from build123d import *

# Parameters (mm, degrees)
F0_R     = 2.25
F1_DEPTH = 1.5


with BuildPart() as f1:
    # F0 (on Top) → F1 (new body)
    with BuildSketch(Plane.XY):
        with BuildLine():
            Line((52.9, 74.5), (-52.9, 74.5))
            ThreePointArc((-52.9, 74.5), (-53.465685, 74.265685), (-53.7, 73.7))
            Line((-53.7, 73.7), (-53.7, 68.7))
            ThreePointArc((-53.7, 68.7), (-56.248171, 62.548171), (-62.4, 60))
            Line((-62.4, 60), (-73.7, 60))
            ThreePointArc((-73.7, 60), (-74.265685, 59.765685), (-74.5, 59.2))
            Line((-74.5, 59.2), (-74.5, -59.2))
            ThreePointArc((-74.5, -59.2), (-74.265685, -59.765685), (-73.7, -60))
            Line((-73.7, -60), (-62.4, -60))
            ThreePointArc((-62.4, -60), (-56.248171, -62.548171), (-53.7, -68.7))
            Line((-53.7, -68.7), (-53.7, -73.7))
            ThreePointArc((-53.7, -73.7), (-53.465685, -74.265685), (-52.9, -74.5))
            Line((-52.9, -74.5), (52.9, -74.5))
            ThreePointArc((52.9, -74.5), (53.465685, -74.265685), (53.7, -73.7))
            Line((53.7, -73.7), (53.7, -68.7))
            ThreePointArc((53.7, -68.7), (56.248171, -62.548171), (62.4, -60))
            Line((62.4, -60), (73.7, -60))
            ThreePointArc((73.7, -60), (74.265685, -59.765685), (74.5, -59.2))
            Line((74.5, -59.2), (74.5, 59.2))
            ThreePointArc((74.5, 59.2), (74.265685, 59.765685), (73.7, 60))
            Line((73.7, 60), (62.4, 60))
            ThreePointArc((62.4, 60), (56.248171, 62.548171), (53.7, 68.7))
            Line((53.7, 68.7), (53.7, 73.7))
            ThreePointArc((53.7, 73.7), (53.465685, 74.265685), (52.9, 74.5))
        make_face()
        with Locations((-48, -69.1)):
            Circle(F0_R, mode=Mode.SUBTRACT)
        with Locations((48, -69.1)):
            Circle(F0_R, mode=Mode.SUBTRACT)
        with Locations((-48, 69.1)):
            Circle(F0_R, mode=Mode.SUBTRACT)
        with Locations((48, 69.1)):
            Circle(F0_R, mode=Mode.SUBTRACT)
    extrude(amount=F1_DEPTH)


solid = f1.part
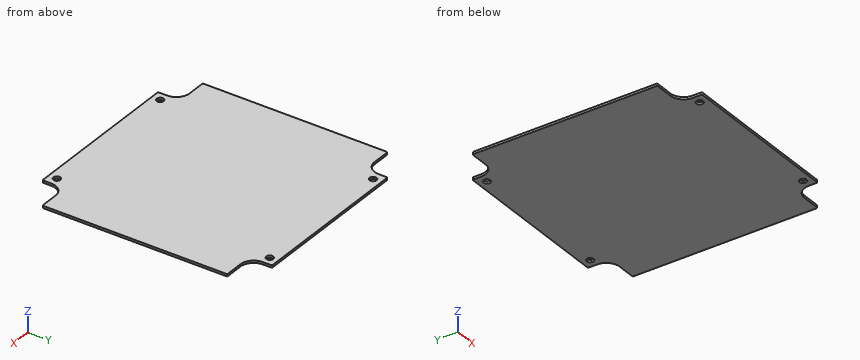
Build history of the part. All positions in model axes, mm. Round coordinates to 2 decimals unless told otherwise and drop trailing zeros. Write each loop counter-clockwise with the first axis right and the second up, starting at its lowest first coordinate (ties: lowest second). Pieces come first, ordered by that corner, then holes. Notation, with made-up numbers: (-24.5, 69) -> (23.5, 69) arc R22 ccw to (23.5, 104) -> close; hole circle Ø1 at (59, 48). An arc over 180 degrees is marked (long way). Use one line per item in the form item = value.
Q1. Drill centre lines: L1, parallel to Y at x = 48, z = 0.5; L2, parallel to Y at x = 53, z = 0.8. Where is each one in solid material? Low to high.
Conclusion:
L1 = -74.5 to -71.35, -66.85 to 66.85, 71.35 to 74.5
L2 = -74.49 to 74.49
Q2. Band-saw the part on A-A, the plane x = -48. Write the cut outline in (y, z).
Conclusion:
outline = (-74.5, 0) -> (-71.35, 0) -> (-71.35, 1.5) -> (-74.5, 1.5) -> close; (-66.85, 0) -> (66.85, 0) -> (66.85, 1.5) -> (-66.85, 1.5) -> close; (71.35, 0) -> (74.5, 0) -> (74.5, 1.5) -> (71.35, 1.5) -> close
Q3. Drop flat-ended pins along their axis: P1, Ø5, axis at x = -48, y = 69.1, coming from the -Z side; P2, Ø0.8, axis at x = 69, z = 1, coming from the +Y side. Give the stop position or say it passes through.
Conclusion:
P1 = 0
P2 = 60
Q4. Band-saw the part on C-C, the plane x = 58. Write the cut outline in (y, z), then the cut area to 3 significant figures.
Conclusion:
outline = (-61.19, 0) -> (61.19, 0) -> (61.19, 1.5) -> (-61.19, 1.5) -> close
area = 184 mm²
Q5. Band-saw the part on B-B, the plane z = 1.2. Write the cut outline in (x, y).
Conclusion:
outline = (-74.5, -59.2) arc R0.8 ccw to (-73.7, -60) -> (-62.4, -60) arc R8.7 cw to (-53.7, -68.7) -> (-53.7, -73.7) arc R0.8 ccw to (-52.9, -74.5) -> (52.9, -74.5) arc R0.8 ccw to (53.7, -73.7) -> (53.7, -68.7) arc R8.7 cw to (62.4, -60) -> (73.7, -60) arc R0.8 ccw to (74.5, -59.2) -> (74.5, 59.2) arc R0.8 ccw to (73.7, 60) -> (62.4, 60) arc R8.7 cw to (53.7, 68.7) -> (53.7, 73.7) arc R0.8 ccw to (52.9, 74.5) -> (-52.9, 74.5) arc R0.8 ccw to (-53.7, 73.7) -> (-53.7, 68.7) arc R8.7 cw to (-62.4, 60) -> (-73.7, 60) arc R0.8 ccw to (-74.5, 59.2) -> close; hole circle Ø4.5 at (-48, -69.1); hole circle Ø4.5 at (-48, 69.1); hole circle Ø4.5 at (48, -69.1); hole circle Ø4.5 at (48, 69.1)
